Model file for the job. Use its own axes, mm. A direction names the side the tool comes from. Give positions to 0.01 mm unless a question says otherwise; leave off trailing zeros. Loops run counter-clockwise (first coordinate to the right, second up) from the corner with the lowest first, then second, coordinate; pieces in that order, holes last. Notation, with made-up numbers: M -40,19 L -5,19 A12 ccw -5,35 Z; hole C 20,9 d6. An arc over 180 degrees is marked long. Answer in a Markdown table with one row per item.
```python
from build123d import *

# Parameters (mm, degrees)
SKETCH1_R                = 1.25
BOSS_EXTRUDE1_DEPTH      = 14
BOSS_EXTRUDE2_DEPTH      = 1
BOSS_EXTRUDE2_DEPTH_BACK = 1
SKETCH3_W                = 11.8
SKETCH3_H                = 3.8
BOSS_EXTRUDE3_DEPTH      = 2


with BuildPart() as part:
    # Sketch1 → Boss-Extrude1 (new body)
    with BuildSketch(Plane(origin=(0, 0, 0), x_dir=(1, 0, 0), z_dir=(0, 1, 0))):
        with Locations(Location((0, 0, 0), (0, 0, 270))):
            Circle(SKETCH1_R)
    extrude(amount=BOSS_EXTRUDE1_DEPTH)

    # Sketch3 → Boss-Extrude2 (add, two sides: drawn at the far end of the back side and taken through both)
    with BuildSketch(Plane(origin=(0, 14, 0), x_dir=(1, 0, 0), z_dir=(0, 1, 0)).offset(-BOSS_EXTRUDE2_DEPTH_BACK)):
        with Locations((1e-09, -0.2)):
            Rectangle(SKETCH3_W, SKETCH3_H)
    extrude(amount=BOSS_EXTRUDE2_DEPTH + BOSS_EXTRUDE2_DEPTH_BACK)

    # Sketch4 → Boss-Extrude3 (add)
    with BuildSketch(Plane(origin=(0, 15, 0), x_dir=(1, 0, 0), z_dir=(0, 1, 0))):
        with BuildLine():
            Line((5.900000001, 1.7), (-5.899999999, 1.7))
            ThreePointArc((-5.899999999, 1.7), (1e-09, 7.6), (5.900000001, 1.7))
        make_face()
    extrude(amount=-BOSS_EXTRUDE3_DEPTH)


solid = part.part
```
(1) Which spindle directions (+Z, -Z, +X, -X, +Y, -Y) get a long thin tool onto all of the face, cutting with end or side? Do faces 1 (the cylindrical face through (-1.22, 6.41, -0.27)), 2 (the flat face through (0, 15, -2)). Say none if no direction does.
Established:
| item | result |
|---|---|
| face 1 | -Y |
| face 2 | +Z, -Z, +X, -X, +Y |
(2) Wall check: L1, parallel to Y at x = -1.75, z = -3.25; L2, parallel to X at y = 10, z = 0; L3, parallel to X at y = 3.25, z = -0.5. Give the ranges that are in metal, low to high.
Established:
| item | result |
|---|---|
| L1 | y = 13 to 15 |
| L2 | x = -1.25 to 1.25 |
| L3 | x = -1.15 to 1.15 |
(3) Saw through at C-C, the plane y = 8.25. Give the cut face in (x, z), and give its area (3 significant figures).
Established:
| item | result |
|---|---|
| outline | C 0,0 d2.5 |
| area | 4.91 mm2 |
(4) Saw through at D-D, the plane z = -5.25. Give the cut face in (x, y), and give its area (3 significant figures).
Established:
| item | result |
|---|---|
| outline | M -4.71,13 L 4.71,13 L 4.71,15 L -4.71,15 Z |
| area | 18.8 mm2 |
(5) Saw through at B-B, the plane z = 0. Give the cut face in (x, y).
Established:
| item | result |
|---|---|
| outline | M -5.9,13 L -1.25,13 L -1.25,0 L 1.25,0 L 1.25,13 L 5.9,13 L 5.9,15 L -5.9,15 Z |
(6) Flat gauge pins, fed straight in: P1, Ø2, axis at x = 2.5, z = -3, coming from the -Y side; P2, Ø4, axis at x = -0.5, y = 8, coming from the +Z side. Where does each tip first touch, or does it go through?
Established:
| item | result |
|---|---|
| P1 | stops at y = 13 |
| P2 | stops at z = 1.25 |
(7) Saw through at A-A, the plane x = 0. Give the cut face in (y, z), and give its area (3 significant figures).
Established:
| item | result |
|---|---|
| outline | M 0,-1.25 L 13,-1.25 L 13,-7.6 L 15,-7.6 L 15,2.1 L 13,2.1 L 13,1.25 L 0,1.25 Z |
| area | 51.9 mm2 |
